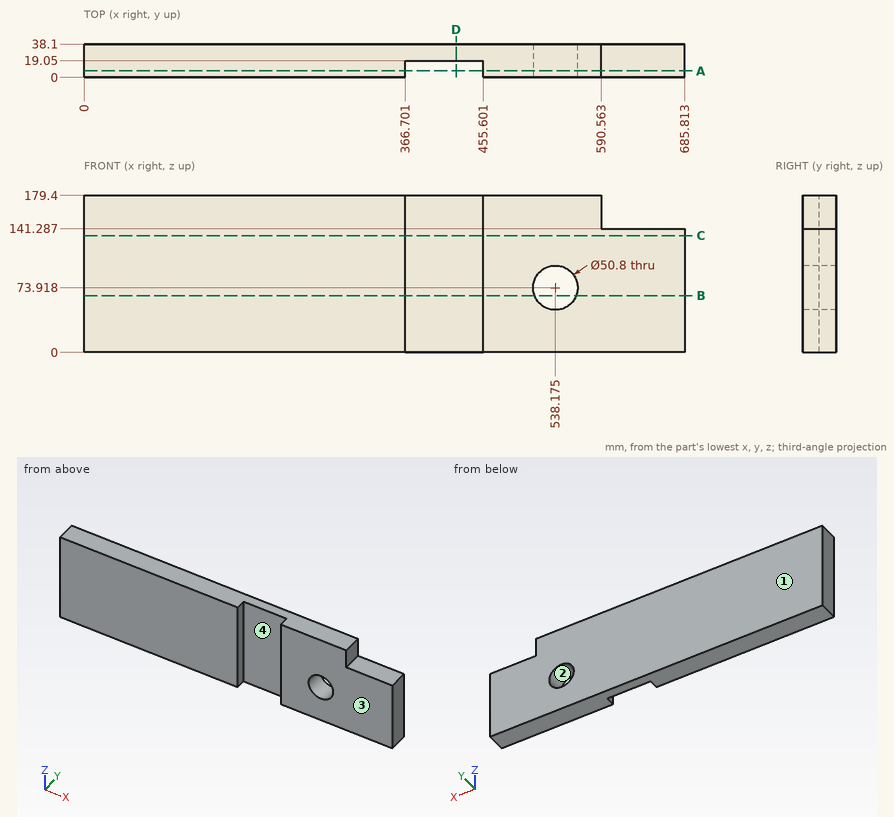
Here's the drawing with two shaded views (mm, measured from the low corner). I have some questions. A direction names the side the tool comes from. Give positions to 0.01 mm unless a question says otherwise; leave off trailing zeros. Write each loop counter-clockwise with the first axis right and the second up, starting at its lowest first coordinate (ties: lowest second). Pieces come first, ordered by that corner, then holes. Notation, with made-up numbers: (58, -31) -> (90, -31) arc R38 cw to (90, 7) -> close; hole circle Ø5 at (-32.5, 0). An arc over 180 degrees is marked (long way). Use one line per item in the form item = value.
1) If I drill on L1, parallel to X at y = 9.5, z = 169; L2, parallel to X at y = 5, z = 19.5; L3, parallel to Y at x = 376.5, z = 97.5, over which ranges is the centre line in solid material (lowest first)? Write a range as [from, to].
Verdict:
L1 = [0, 366.7], [455.6, 590.56]
L2 = [0, 366.7], [455.6, 685.81]
L3 = [19.05, 38.1]
2) Suppose I cut it at A-A (y = 7.5). Please give me the cut outline in (x, z) (1 decimal), and give its area (3 significant figures).
Verdict:
outline = (0, 0) -> (366.7, 0) -> (366.7, 179.4) -> (0, 179.4) -> close; (455.6, 0) -> (685.8, 0) -> (685.8, 141.3) -> (590.6, 141.3) -> (590.6, 179.4) -> (455.6, 179.4) -> close; hole circle Ø50.8 at (538.2, 73.9)
area = 101,000 mm2
3) On a 3-axis mill with a long thin cutter (end or side, diameter ignored), from which of +Z, -Z, +X, -X, +Y, -Y can I reach the whole of each face in a straight line? I mean the marked faces 3 and 4. Say none if no direction works.
Verdict:
face_3 = +Z, -Z, +X, -X, -Y
face_4 = +Z, -Z, -Y
4) We'd pull the mould along Z, two halves only. Please class the marked faces 1 and 2: +Z half, -Z half, draft (parallel to the pull), parting line (faces both ways), or undercut.
Verdict:
face_1 = draft
face_2 = undercut
5) Suppose I cut it at D-D (x = 425). Please give me the cut outline in (y, z).
Verdict:
outline = (19.05, 0) -> (38.1, 0) -> (38.1, 179.4) -> (19.05, 179.4) -> close
6) Suppose I cut it at C-C (z = 133.5). Please give me the cut outline in (x, y).
Verdict:
outline = (0, 0) -> (366.7, 0) -> (366.7, 19.05) -> (455.6, 19.05) -> (455.6, 0) -> (685.81, 0) -> (685.81, 38.1) -> (0, 38.1) -> close
7) Suppose I cut it at B-B (z = 65). Please give me the cut outline in (x, y).
Verdict:
outline = (0, 0) -> (366.7, 0) -> (366.7, 19.05) -> (455.6, 19.05) -> (455.6, 0) -> (514.39, 0) -> (514.39, 38.1) -> (0, 38.1) -> close; (561.96, 0) -> (685.81, 0) -> (685.81, 38.1) -> (561.96, 38.1) -> close
8) I'm going to push flat-ended pins straight in: pin 1 (3 mm diameter, centred on x = 442, z = 120, fed in from -Y); pin 2 (19 mm diameter, centred on y = 18.5, z = 156.5, fed in from +X). Where does each tip first touch, or does it pass through?
Verdict:
pin_1 = 19.05
pin_2 = 590.56
